Design review of the part shown in the three views and the two pictorial views. Dimensions are in mm from the part's minimum x, y and z. A direction names the side the tool comes from. Coordinates: 2 decimals unless noted, no trailing zeros. Loops run counter-clockwise (first coordinate to the right, second up) from the corner with the lowest first, then second, coordinate; pieces in that order, holes last. Notation, with made-up numbers: (13, -6) -> (20, -6) arc R18 cw to (20, 17) -> close; hole circle Ø7 at (56, 2). An arc over 180 degrees is marked (long way). Answer in a Markdown table with one row per item.
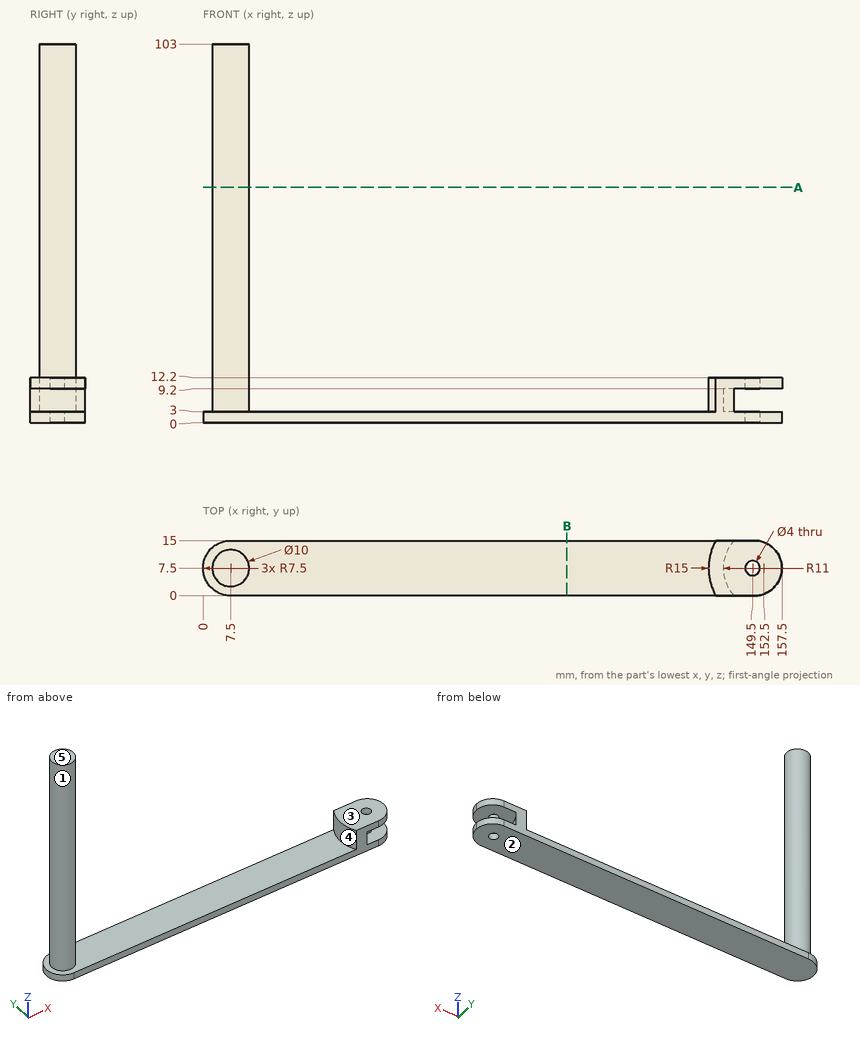
Item 1: For the marked faces 1, 2 and 3, list the 3-axis set-ups (+Z, -Z, +X, -X, +Y, -Y) from which the entire face can be reached by the end or side of a thin tool; tool diameter is ignored.
Worked answers:
| item | result |
|---|---|
| face 1 | +Z |
| face 2 | -Z, +X, -X, +Y, -Y |
| face 3 | +Z, +X, +Y, -Y |
Item 2: Take a section at B-B, the plane x = 99. State the section outline as (y, z) points.
Worked answers:
| item | result |
|---|---|
| outline | (0, 0) -> (15, 0) -> (15, 3) -> (0, 3) -> close |
Item 3: Take a section at A-A, the plane z = 64. State the section outline as (x, y) points, and give its area (3 significant figures).
Worked answers:
| item | result |
|---|---|
| outline | circle Ø10 at (7.5, 7.5) |
| area | 78.5 mm² |
Item 4: Insertion check: pin 1 (1 mm diameter, centred on y = 3, z = 77.5, fed in from +X); pin 2 (1.5 mm diameter, centred on x = 80.5, y = 4.5, fed in from +Z); pin 3 (2.5 mm diameter, centred on x = 149.5, y = 7.5, fed in from +Z); pin 4 (4 mm diameter, centred on y = 8, z = 26.5, fed in from -X). Each pin has a flat end and moves straight along its axis. Give the tip position at first contact, or say it passes through.
Worked answers:
| item | result |
|---|---|
| pin 1 | x = 10.5 |
| pin 2 | z = 3 |
| pin 3 | through |
| pin 4 | x = 2.5 |
Item 5: For L1, parallel to Y at x = 149.5, z = 1.05; L2, parallel to X at y = 8, z = 69.5 (3 decimals); L3, parallel to Z at x = 83.5, y = 7.75, list the stretches that pass through material, from the lowest coordinate up.
Worked answers:
| item | result |
|---|---|
| L1 | 0 to 5.5, 9.5 to 15 |
| L2 | 2.525 to 12.475 |
| L3 | 0 to 3 |
Item 6: The part is to be moulded in two halves that separate along X. For the marked faces 4 and 5, say which applies: +X half, -X half, draft (parallel to the pull), parting line (faces both ways), or undercut.
Worked answers:
| item | result |
|---|---|
| face 4 | undercut |
| face 5 | draft |
